Can you work these out from the drawing? Everything is in mm from the part's minimum corner. A direction names the side the tool comes from. Give positions to 0.01 mm unless a question says otherwise; leave off trailing zeros. Write each loop counter-clockwise with the first axis right and the second up, starting at its lowest first coordinate (ties: lowest second). Pieces come first, ordered by that corner, then holes. Notation, with made-up numbers: (78.5, 40.25) -> (125.5, 40.25) arc R30 ccw to (125.5, 68.25) -> close; hole circle Ø8 at (-26, 4.5). An arc over 180 degrees is marked (long way). Use one line per item in the form item = value.
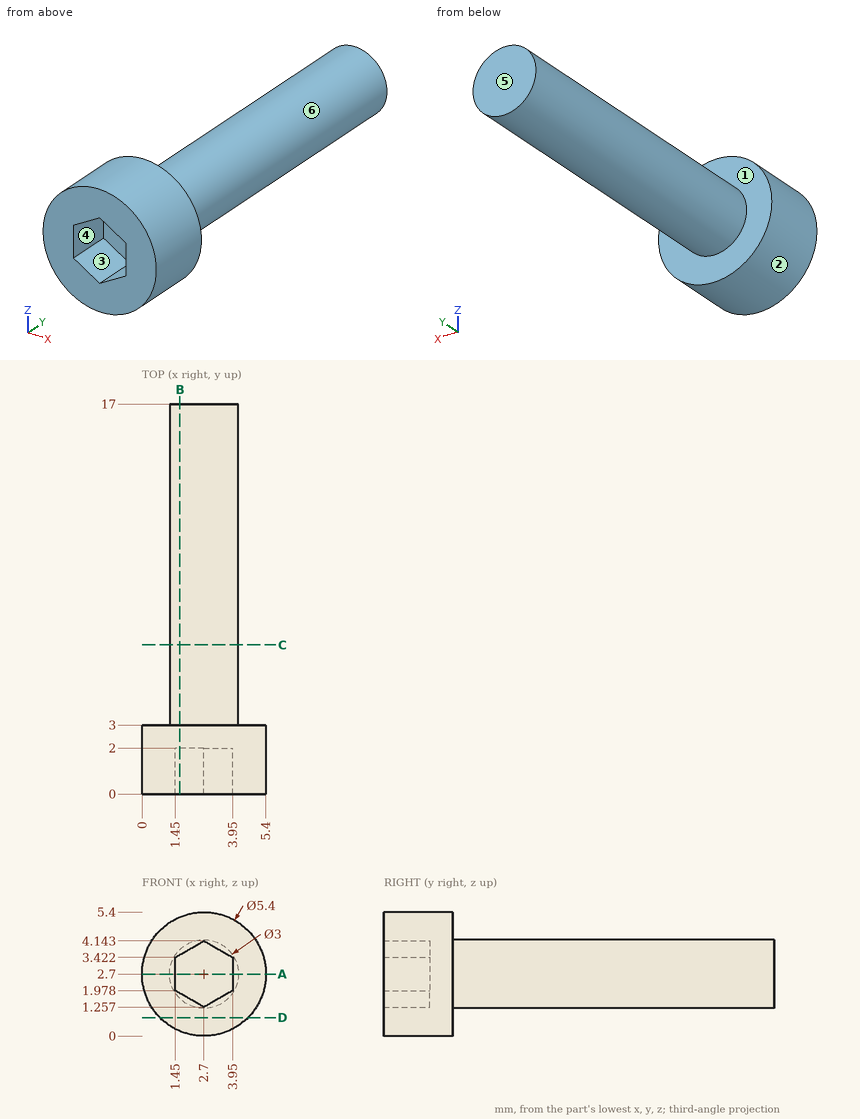
Q1. I want a section at D-D, the plane z = 0.8. Write out the boundary of the cut face in (x, y).
Result set:
outline = (0.78, 0) -> (4.62, 0) -> (4.62, 3) -> (0.78, 3) -> close
Q2. Will these pins go through, and if not, where does the flat tip stop? pin 1 Ø1 at (x, y) = (1, 9.5) entering from -Z; pin 2 Ø2 at (x, y) = (1, 9) entering from -Z; pin 3 Ø3 at (y, z) = (6, 3) entering from -X.
Result set:
pin_1 = 1.8
pin_2 = 1.37
pin_3 = 1.2
Q3. I want a section at C-C, the plane y = 6.5. Write out the boundary of the cut face in (x, z).
Result set:
outline = circle Ø3 at (2.7, 2.7)
Q4. If I drill on line 1 along Y through (x, z) = (4.2, 0.55); line 2 along Y through (x, z) = (1.9, 3.3); line 3 along Z through (x, y) = (2.75, 10.75), over which ranges is the centre line in solid material (lowest first)? Write a range as from..to.
Result set:
line_1 = 0..3
line_2 = 2..17
line_3 = 1.2..4.2
Q5. If we mould it in two halves opening along X, with no side actions, what happens to the marked faces 3, 4, 5 and 6? For each: +X half, -X half, draft (parallel to the pull), parting line (faces both ways), or undercut.
Result set:
face_3 = undercut
face_4 = undercut
face_5 = draft
face_6 = parting line
Q6. Which directions (+Z, -Z, +X, -X, +Y, -Y) give clear straight access to the entire face, cutting with the end or side of a thin tool? Please do the marked faces 1 and 2.
Result set:
face_1 = +Y
face_2 = +Y, -Y
Q7. I want a section at A-A, the plane z = 2.7. Write out the boundary of the cut face in (x, y), and give its area (3 significant figures).
Result set:
outline = (0, 0) -> (1.45, 0) -> (1.45, 2) -> (3.95, 2) -> (3.95, 0) -> (5.4, 0) -> (5.4, 3) -> (4.2, 3) -> (4.2, 17) -> (1.2, 17) -> (1.2, 3) -> (0, 3) -> close
area = 53.2 mm2
Q8. I want a section at B-B, the plane x = 1.65. Write out the boundary of the cut face in (y, z).
Result set:
outline = (0, 0.21) -> (3, 0.21) -> (3, 1.63) -> (17, 1.63) -> (17, 3.77) -> (3, 3.77) -> (3, 5.19) -> (0, 5.19) -> (0, 3.54) -> (2, 3.54) -> (2, 1.86) -> (0, 1.86) -> close
